Design review of the part shown in the three views and the two pictorial views. Dimensions are in mm from the part's minimum x, y and z. A direction names the side the tool comes from. Coordinates: 2 decimals unless noted, no trailing zeros. Write each loop counter-clockwise with the first axis right and the second up, starting at its lowest first coordinate (ties: lowest second). Pieces come first, ordered by that corner, then holes. Notation, with made-up numbers: (35.25, 87.25) -> (79.25, 87.25) arc R21 ccw to (79.25, 124.25) -> close; hole circle Ø2 at (49.5, 62.25). An arc over 180 degrees is marked (long way). Answer in a Markdown table with one row per item. Add a question column.
Item 1: Take a section at B-B, the plane x = 15. Write out the cut boundary in (y, z), and give its area (4 significant figures).
Item 2: Draft analysis for pull direction Y (two halves, no side actions). For the marked faces 3, 4 and 5, state which applies: released by +Y, released by -Y, zero draft, split by the parting line, or undercut.
Item 3: Take a section at C-C, the plane z = 4.25. Write out the cut boundary in (x, y).
Item 4: For the marked faces 1 and 2, list the 3-axis set-ups (+Z, -Z, +X, -X, +Y, -Y) from which the entire face can be reached by the end or side of a thin tool; tool diameter is ignored.
Item 5: To check wall thickness, follow line 1 (Y direction, x = 15, z = 14.1); line 2 (X direction, y = 26.5, z = 3); line 3 (Y direction, x = 16.5, z = 7.75). State the ranges of each line that lie inside material, in increasing order.
Item 6: Clearance check with a flat-ended pin moving along its axis: P1, Ø17, axis at x = 15, y = 26, coming from the +Z side. State where the tip first meets the part, or that it passes through.
Item 7: Take a section at A-A, the plane z = 14. Write out the cut boundary in (x, y).
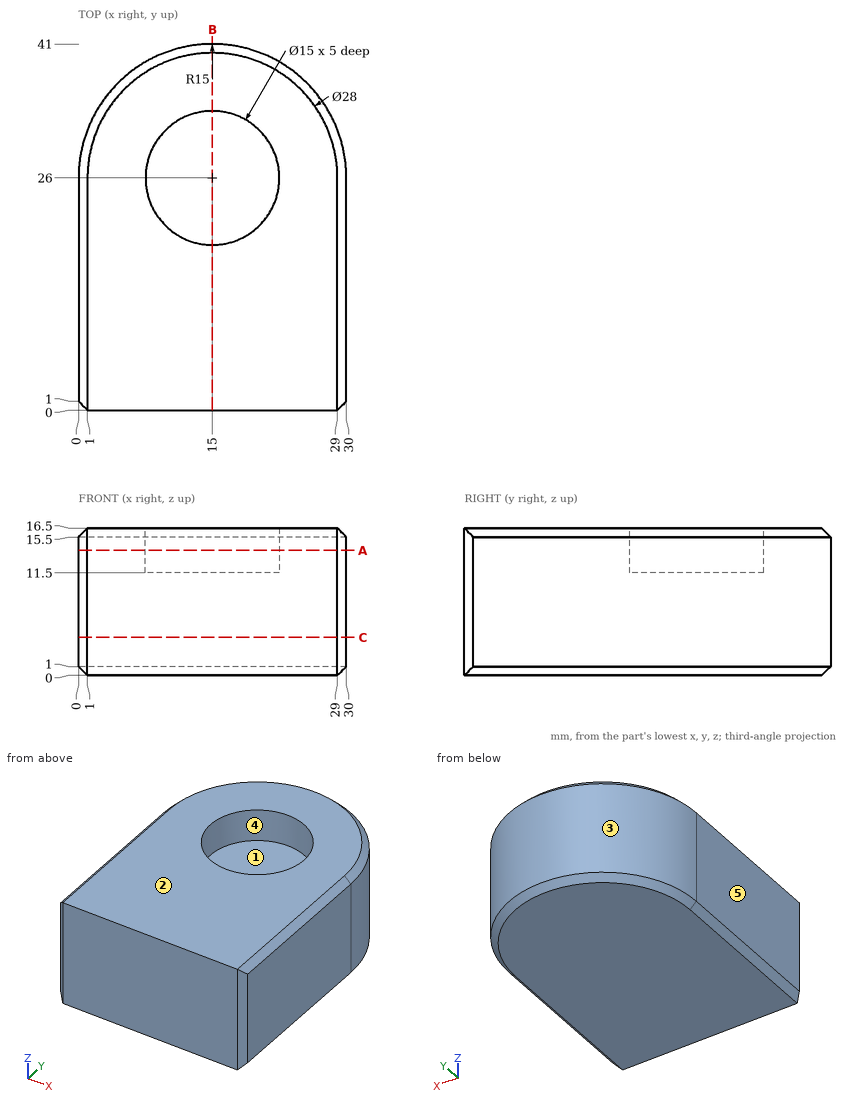
Answers:
| question | item | result |
|---|---|---|
| 1 | outline | (0, 0) -> (40, 0) -> (41, 1) -> (41, 15.5) -> (40, 16.5) -> (33.5, 16.5) -> (33.5, 11.5) -> (18.5, 11.5) -> (18.5, 16.5) -> (0, 16.5) -> close |
| 1 | area | 600.5 mm^2 |
| 2 | face 3 | released by +Y |
| 2 | face 4 | undercut |
| 2 | face 5 | zero draft |
| 3 | outline | (0, 1) -> (1, 0) -> (29, 0) -> (30, 1) -> (30, 26) arc R15 ccw to (0, 26) -> close |
| 4 | face 1 | +Z |
| 4 | face 2 | +Z, +X, -X, +Y, -Y |
| 5 | line 1 | y = 0 to 18.5, 33.5 to 41 |
| 5 | line 2 | x = 0.01 to 29.99 |
| 5 | line 3 | y = 0 to 40.92 |
| 6 | P1 | stops at z = 16.5 |
| 7 | outline | (0, 1) -> (1, 0) -> (29, 0) -> (30, 1) -> (30, 26) arc R15 ccw to (0, 26) -> close; hole circle Ø15 at (15, 26) |
